```python
from build123d import *

# Parameters (mm, degrees)
F0_W     = 56.3245862722
F0_H     = 11.1567229033
F4_DEPTH = 11.1567229033


with BuildPart() as f2:
    # F2: sweep along a path in F1
    with BuildLine(Plane.XY) as f2_path:
        ThreePointArc((-23.6530322582, -43.8611544669), (-13.0490165439, -22.6514177551), (-6.0339360498, 0))
    # F0 (on Front) → F2 (sweep)
    with BuildSketch(Plane.XZ):
        with Locations((1.150039956, 5.5783614516)):
            Rectangle(F0_W, F0_H)
    sweep(path=f2_path.line)

    # F3: sweep along a path in F1
    with BuildLine(Plane.XY) as f3_path:
        ThreePointArc((-6.0339360498, 0), (4.5287353952, -22.758853007), (18.1018076837, -43.8611544669))
    # F0 (on Front) → F3 (sweep)
    with BuildSketch(Plane.XZ):
        with Locations((1.150039956, 5.5783614516)):
            Rectangle(F0_W, F0_H)
    sweep(path=f3_path.line)

    # F1 (on Top) → F4 (join, through all)
    with BuildSketch(Plane.XY):
        with BuildLine():
            ThreePointArc((16.3831246193, 0), (-19.3757451039, 18.0144591983), (-12.569889783, -21.4430855485))
            ThreePointArc((-12.569889783, -21.4430855485), (-8.8880028651, -10.8477045125), (-6.0339360498, 0))
            ThreePointArc((-6.0339360498, 0), (-1.7021386375, -10.3433289498), (3.2543247609, -20.402274877))
            ThreePointArc((3.2543247609, -20.402274877), (12.8173253821, -12.1307275738), (16.3831246193, 0))
        make_face()
    extrude(amount=F4_DEPTH)


solid = f2.part
```
Here's how the part is built. I have some questions about the finished solid (model axes, mm). A direction names the side the tool comes from. Give positions to 0.01 mm unless a question says otherwise; leave off trailing zeros. Loops run counter-clockwise (first coordinate to the right, second up) from the corner with the lowest first, then second, coordinate; pieces in that order, holes last. Notation, with made-up numbers: (2.5, 60.25) -> (55.5, 60.25) arc R22 ccw to (55.5, 75.25) -> close; hole circle Ø8 at (14.25, 69.25). An arc over 180 degrees is marked (long way). Use one line per item in the form item = value. Start each with the question number.
1) For P1, Ø5.5, axis at x = 23, z = 5.5, coming from the +Y side; P2, Ø8, axis at x = 39, y = -11.5, coming from the -Z side; P3, Ø5, axis at y = 5, z = 7.5, coming from the +X side; P4, Ø1.5, axis at x = -6, z = 7, coming from the -Y side, each with a flat end and sliding along its axis, tell me the tip position at first contact or that it passes through.
2) Please list where these lines run through material, in increasing order: line 1 along Y through (x, z) = (26.5, 7); line 2 along Y through (x, z) = (-8, 7); line 3 along X through (y, z) = (-14, 4).
3) Imagine slicing it at A-A (z = 9.5). Please give me the cut outline in (x, y), then the cut area to 3 significant figures.
4) Imagine slicing it at B-B (y = -11). Please give me the cut outline in (x, z).
5) Imagine slicing it at C-C (x = -23). Please give me the cut outline in (y, z), then the cut area to 3 significant figures.
6) Which directions (+Z, -Z, +X, -X, +Y, -Y) give clear straight access to the entire face, cutting with the end or side of a thin tool? Please do faces 1 (the face through (4, -16, 11.157)), 2 (the face through (23, 0, 6)).
Check values:
q1.P1 = 0
q1.P2 = 0
q1.P3 = 16.24
q1.P4 = -50.09
q2.line_1 = -41.5 to 0
q2.line_2 = -49.16 to 22.33
q2.line_3 = -31.56 to 37.02
q3.outline = (-43.52, -37.13) -> (9.83, -55.2) arc R180.05 ccw to (15.16, -44.69) -> (52.13, -34.29) arc R150.74 cw to (29.31, 0) -> (16.38, 0) arc R22.42 ccw (long way) to (-28.1, -3.93) arc R124.99 cw to start
q3.area = 4,200 mm^2
q4.outline = (-30.43, 0) -> (35.2, 0) -> (35.2, 11.16) -> (-30.43, 11.16) -> close
q5.outline = (-44.08, 0) -> (14.65, 0) -> (14.65, 11.16) -> (-44.08, 11.16) -> close
q5.area = 655 mm^2
q6.face_1 = +Z, +X, -X, +Y, -Y
q6.face_2 = +Z, -Z, +X, +Y
